Drawing for the job (mm, zero at the part's lowest x, y, z). A direction names the side the tool comes from. Coordinates: 2 decimals unless noted, no trailing zeros. Order: outer loops, then holes, each group sorted by start corner. A loop starts at its lowest first (then second) coordinate and runs counter-clockwise, first axis right, second up. Notation, with made-up numbers: (-15.75, 37) -> (-0.75, 37) arc R32 ccw to (-0.75, 69) -> close; hole circle Ø6 at (3, 18). An arc over 180 degrees is marked (long way). Write each question's results on one line, items separated by ' | '.
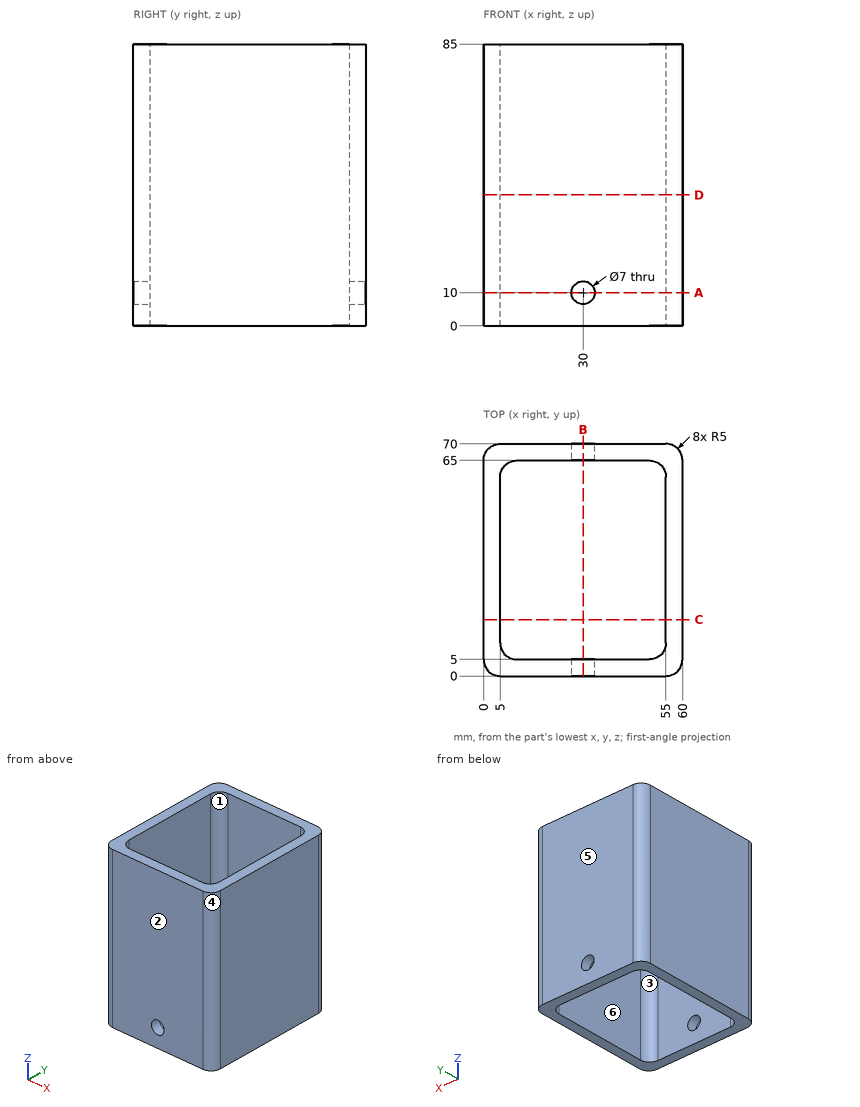
Item 1: Slice it at D-D, the plane z = 39.5. List the corners of the cut face in (x, y).
Answer:
outline: (0, 5) arc R5 ccw to (5, 0) -> (55, 0) arc R5 ccw to (60, 5) -> (60, 65) arc R5 ccw to (55, 70) -> (5, 70) arc R5 ccw to (0, 65) -> close; hole (5, 10) arc R5 ccw to (10, 5) -> (50, 5) arc R5 ccw to (55, 10) -> (55, 60) arc R5 ccw to (50, 65) -> (10, 65) arc R5 ccw to (5, 60) -> close
Item 2: Tool access for the marked faces 1 and 2: list every direction of +Z, -Z, +X, -X, +Y, -Y with a clear straight run to the whole face (end or side of a thin tool).
Answer:
face 1: +Z, -Z | face 2: +Z, -Z, +X, -X, -Y
Item 3: Slice it at A-A, the plane z = 10. List the corners of the cut face in (x, y), and give its area (3 significant figures).
Answer:
outline: (0, 5) arc R5 ccw to (5, 0) -> (26.5, 0) -> (26.5, 5) -> (10, 5) arc R5 cw to (5, 10) -> (5, 60) arc R5 cw to (10, 65) -> (26.5, 65) -> (26.5, 70) -> (5, 70) arc R5 ccw to (0, 65) -> close; (33.5, 0) -> (55, 0) arc R5 ccw to (60, 5) -> (60, 65) arc R5 ccw to (55, 70) -> (33.5, 70) -> (33.5, 65) -> (50, 65) arc R5 cw to (55, 60) -> (55, 10) arc R5 cw to (50, 5) -> (33.5, 5) -> close | area: 1,130 mm^2
Item 4: Pin check, flat tip, straight feed: pin 1 (6.5 mm diameter, centred on x = 30, z = 10, fed in from -Y). Stop position of the tip, or through.
Answer:
pin 1: passes through
Item 5: Pull direction Y, two halves, no side cores. Call the marked faces 3, 4, 5 and 6: released by +Y, released by -Y, zero draft, split by the parting line, or undercut.
Answer:
face 3: undercut | face 4: released by -Y | face 5: released by +Y | face 6: undercut
Item 6: Slice it at C-C, the plane y = 17. List the corners of the cut face in (x, z).
Answer:
outline: (0, 0) -> (5, 0) -> (5, 85) -> (0, 85) -> close; (55, 0) -> (60, 0) -> (60, 85) -> (55, 85) -> close
Item 7: Drill centre lines: line 1 (Z direction, x = 30, y = 1); line 2 (X direction, y = 39.5, z = 36.5); line 3 (Y direction, x = 11, z = 12.5). Where is each one in solid material? Low to high. Write a range as from..to.
Answer:
line 1: z = 0..6.5, 13.5..85 | line 2: x = 0..5, 55..60 | line 3: y = 0..5, 65..70
Item 8: Slice it at B-B, the plane x = 30. List the corners of the cut face in (y, z), and give its area (3 significant figures).
Answer:
outline: (0, 0) -> (5, 0) -> (5, 6.5) -> (0, 6.5) -> close; (0, 13.5) -> (5, 13.5) -> (5, 85) -> (0, 85) -> close; (65, 0) -> (70, 0) -> (70, 6.5) -> (65, 6.5) -> close; (65, 13.5) -> (70, 13.5) -> (70, 85) -> (65, 85) -> close | area: 780 mm^2
